Autodesk Inventor part; units mm, degrees
ref_plane "YZ Plane" through (0, 0, 0) normal (1, 0, 0) x (0, 1, 0)
ref_plane "XZ Plane" through (0, 0, 0) normal (0, 1, 0) x (-1, 0, 0)
ref_plane "XY Plane" through (0, 0, 0) normal (0, 0, 1) x (1, 0, 0)
sketch "Sketch1" plane through (0, 0, 0) normal (0, 0, 1) x (1, 0, 0)
  line L0 (-60.259, 41.2953) -> (59.741, 41.2953)
  line L1 (59.741, 41.2953) -> (59.741, -8.7047)
  line L2 (59.741, -8.7047) -> (-60.259, -8.7047)
  line L3 (-60.259, -8.7047) -> (-60.259, 41.2953)
  dimension "d0" = 120
  dimension "d1" = 50
extrude "Plate1" add sketch "Sketch1" along normal blind 0.5
sketch "Sketch2" plane through (0, 0, 0.5) normal (0, 0, 1) x (1, 0, 0)
  line L0 (3.7677, 16.6653) -> (23.7677, 16.6653)
  line L1 (23.7677, 16.6653) -> (23.7677, 8.6653)
  line L2 (23.7677, 8.6653) -> (3.7677, 8.6653)
  line L3 (3.7677, 8.6653) -> (3.7677, 16.6653)
  point P0 (13.7677, 12.6653)
  point P1 (13.7677, 12.6653)
  dimension "LG_G" = 20
  dimension "LT_G" = 8
  dimension "d5" = 10
  dimension "d6" = 4
extrude "Extrusion1" add sketch "Sketch2" against normal blind 1.5
sketch "Sketch3" plane through (0, 0, 0.5) normal (0, 0, 1) x (1, 0, 0)
  line L0 (3.7677, 16.6653) -> (23.7677, 16.6653)
  line L1 (3.7677, 8.6653) -> (3.7677, 16.6653)
  line L2 (23.7677, 8.6653) -> (3.7677, 8.6653)
  line L3 (23.7677, 16.6653) -> (23.7677, 8.6653)
  line L4 (4.2677, 16.6653) -> (23.2677, 16.6653)
  line L5 (23.2677, 16.6653) -> (23.2677, 8.6653)
  line L6 (23.2677, 8.6653) -> (4.2677, 8.6653)
  line L7 (4.2677, 8.6653) -> (4.2677, 16.6653)
  dimension "d9" = 0.5
  dimension "d10" = 0.5
extrude "Extrusion2" cut sketch "Sketch3" against normal blind 1 contours L0 L5 L2 L7
sketch "Sketch4" plane through (0, 0, 0.5) normal (0, 0, 1) x (1, 0, 0)
  line L0 (4.2677, 16.6653) -> (23.2677, 16.6653)
  line L1 (23.2677, 8.6653) -> (4.2677, 8.6653)
  line L2 (4.2677, 16.6653) -> (23.2677, 16.6653)
  line L3 (4.2677, 8.6653) -> (4.2677, 16.6653)
  line L4 (23.2677, 8.6653) -> (4.2677, 8.6653)
  line L5 (23.2677, 16.6653) -> (23.2677, 8.6653)
  line L6 (3.7677, 17.1653) -> (23.7677, 17.1653)
  line L7 (23.7677, 17.1653) -> (23.7677, 16.6653)
  line L8 (23.7677, 16.6653) -> (3.7677, 16.6653)
  line L9 (3.7677, 16.6653) -> (3.7677, 17.1653)
  line L10 (3.7677, 8.6653) -> (23.7677, 8.6653)
  line L11 (23.7677, 8.6653) -> (23.7677, 8.1653)
  line L12 (23.7677, 8.1653) -> (3.7677, 8.1653)
  line L13 (3.7677, 8.1653) -> (3.7677, 8.6653)
  dimension "d13" = 0.5
  dimension "d14" = 0.5
  dimension "d15" = 0.5
  dimension "d16" = 0.5
extrude "Cut1" cut sketch "Sketch4" against normal blind 0.5 contours L8 L9 L6 L7 L0 | L1 L10 L11 L12 L13
equation "\"d7\" = 3 * Thickness"
equation "\"d9\" = Thickness"
equation "\"d10\" = Thickness"
equation "\"d11\" = 2 * Thickness"
equation "\"d13\" = Thickness"
equation "\"d14\" = Thickness"
equation "\"d15\" = Thickness"
equation "\"d16\" = Thickness"
equation "\"d17\" = Thickness"
equation "\"d2\" = Thickness"
equation "\"BendRadius\" = Thickness"
equation "\"BendReliefWidth\" = Thickness"
equation "\"BendReliefDepth\" = 0.5 * Thickness"
equation "\"CornerReliefSize\" = 4 * Thickness"
equation "\"MinimumRemnant\" = 2 * Thickness"
equation "\"TransitionRadius\" = BendRadius"
equation "\"JacobiRadiusSize\" = BendRadius"
equation "\"GapSize\" = Thickness"
properties part number "Ambutisare1"
Source: CAD feature listing. Evaluate the final solid. Frame: model axes, mm. A direction names the side the tool comes from. Give positions to 0.01 mm unless a question says otherwise; leave off trailing zeros. Write each loop counter-clockwise with the first axis right and the second up, starting at its lowest first coordinate (ties: lowest second). Pieces come first, ordered by that corner, then holes. Notation, with made-up numbers: M -35.5,24 L 12.5,24 A30 cw 12.5,48 Z; hole C 1,64 d4. An arc over 180 degrees is marked long. Answer as a JSON object with one key per item and string values.
Q1. Contact query for flat-ended pins moving along their axis: P1, Ø0.5, axis at y = 12.5, z = -0.5, coming from the +X side; P2, Ø15, axis at x = -4, y = 12, coming from the -Z side. Output: stop coordinate, or through.
Geometry check:
{"P1": "stops at x = 23.77", "P2": "stops at z = 0"}
Q2. Cut plane A-A, the plane x = 19. Return the cut outline in (y, z), then the cut area to 3 significant figures.
Geometry check:
{"outline": "M -8.7,0 L 8.17,0 L 8.17,0.5 L -8.7,0.5 Z; M 8.67,-1 L 16.67,-1 L 16.67,-0.5 L 8.67,-0.5 Z; M 17.17,0 L 41.3,0 L 41.3,0.5 L 17.17,0.5 Z", "area": "24.5 mm^2"}
Q3. Cut plane B-B, the plane y = 29. Return the cut outline in (x, z), then the cut area to 3 significant figures.
Geometry check:
{"outline": "M -60.26,0 L 59.74,0 L 59.74,0.5 L -60.26,0.5 Z", "area": "60.0 mm^2"}
Q4. Access query for faces 1 (the face through (14, 13, -0.5)), 2 (the face through (-1, 17, 0.5)). Directions: +Z, -Z, +X, -X, +Y, -Y. A direction counts if a zero-diameter tool reaches every point of the face in a straight line with its end or side. Return the directions, or none.
Geometry check:
{"face 1": "+Z, +Y, -Y", "face 2": "+Z, +X, -X, +Y, -Y"}
Q5. Ray query, line 1 along Y through (x, z) = (15, 0.2); line 2 along Z through (x, y) = (-46.5, 14); line 3 along X through (y, z) = (9.5, -0.3). Return the intervals inside material, ascending.
Geometry check:
{"line 1": "y = -8.7 to 8.17, 17.17 to 41.3", "line 2": "z = 0 to 0.5", "line 3": "x = 3.77 to 4.27, 23.27 to 23.77"}
